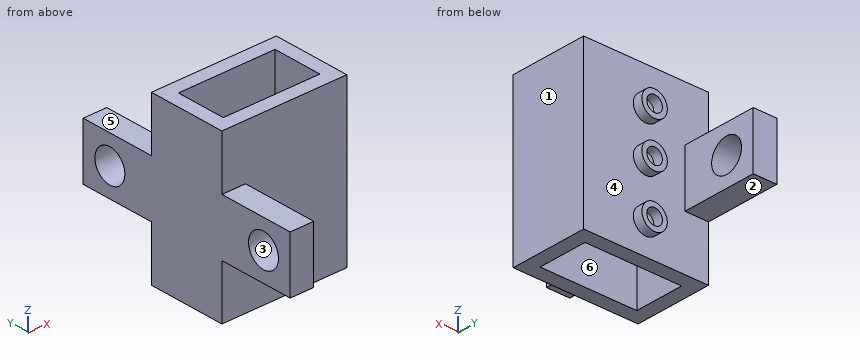
from build123d import *

# Parameters (mm, degrees)
F0_W      = 26.5
F0_H      = 35
F1_DEPTH  = 16.5
F2_W      = 20.5
F2_H      = 10.5
F3_DEPTH  = 35
F4_R      = 2.7
F4_R_2    = 1.65
F5_DEPTH  = 2
F6_W      = 5
F6_H      = 12
F7_DEPTH  = 16
F8_W      = 5
F8_H      = 12
F9_DEPTH  = 16
F10_R     = 3.5
F11_DEPTH = 5
F12_R     = 3.5
F13_DEPTH = 5


with BuildPart() as f1:
    # F0 (on Front) → F1 (new body)
    with BuildSketch(Plane.XZ):
        Rectangle(F0_W, F0_H)
    extrude(amount=F1_DEPTH)

    # F2 (on face) → F3 (cut)
    with BuildSketch(Plane.XY.offset(17.5)):
        with Locations((0, -8.25)):
            Rectangle(F2_W, F2_H)
    extrude(amount=-F3_DEPTH, mode=Mode.SUBTRACT)

    # F4 (on face) → F5 (join)
    with BuildSketch(Plane(origin=(0, 0, 0), x_dir=(-1, 0, 0), z_dir=(0, 1, 0))):
        Circle(F4_R)
        Circle(F4_R_2, mode=Mode.SUBTRACT)
        with Locations((0, 9.5)):
            Circle(F4_R)
        with Locations((0, 9.5)):
            Circle(F4_R_2, mode=Mode.SUBTRACT)
        with Locations((0, -11)):
            Circle(F4_R)
        with Locations((0, -11)):
            Circle(F4_R_2, mode=Mode.SUBTRACT)
    extrude(amount=F5_DEPTH)

    # F6 (on face) → F7 (join)
    with BuildSketch(Plane.XZ.offset(16.5)):
        with Locations((-10.75, 0)):
            Rectangle(F6_W, F6_H)
    extrude(amount=F7_DEPTH)

    # F8 (on face) → F9 (join)
    with BuildSketch(Plane(origin=(0, 0, 0), x_dir=(-1, 0, 0), z_dir=(0, 1, 0))):
        with Locations((10.75, 0)):
            Rectangle(F8_W, F8_H)
    extrude(amount=F9_DEPTH)

    # F10 (on face) → F11 (cut)
    with BuildSketch(Plane.YZ.offset(-8.25)):
        with Locations((9.75, 0)):
            Circle(F10_R)
    extrude(amount=-F11_DEPTH, mode=Mode.SUBTRACT)

    # F12 (on face) → F13 (cut)
    with BuildSketch(Plane.YZ.offset(-8.25)):
        with Locations((-26.25, 0)):
            Circle(F12_R)
    extrude(amount=-F13_DEPTH, mode=Mode.SUBTRACT)


solid = f1.part
Input: part model. Units: mm. Frame: model coordinates. Face numbers are marked on the shaded views. A direction names the side the tool comes from. Coordinates: 2 decimals unless noted, no trailing zeros. Write each loop counter-clockwise with the first axis right and the second up, starting at its lowest first coordinate (ties: lowest second). Pieces come first, ordered by that corner, then holes. Notation, with made-up numbers: M 6.25,30 L 23.25,30 A23 cw 23.25,69 Z; hole C -14.5,39 d7. An arc over 180 degrees is marked long. Answer as a JSON object with one key per item and string values. Group by question number.
(1) Section A-A on x = -9. Output: boundary loops of the cut face in (y, z), plus the area to 3 significant figures.
(2) Section B-B on z = 1. Output: boundary loops of the cut face in (x, y), plus the area to 3 significant figures.
(3) Mould query, pull axis Z, two halves, no side actions, for the marked faces 1, 2 and 3. Classes: pulls with the +Z half, pulls with the -Z half, needs draft (parallel to the pull), parting line crosses it, or undercut.
(4) Ray query, line 1 along Z through (x, y) = (0, 1.2); line 2 along Z through (x, y) = (-11.85, 9.75); line 3 along Y through (x, z) = (0, 4). Return the intervals inside material, ascending. Write a range as [from, to].
(5) Section D-D on x = -5.25. Output: boundary loops of the cut face in (y, z).
(6) Set-up query: the marked faces 4, 5 and 6. Return all of +Z, -Z, +X, -X, +Y, -Y with unobstructed straight access to the full face (end or side cutting, diameter ignored); none if empty.
(7) Section C-C on y = -9.5. Output: boundary loops of the cut face in (x, z).
(8) Contact query for flat-ended pins moving along their axis: P1, Ø4, axis at x = 10.5, z = 2, coming from the +Y side; P2, Ø5.5, axis at x = -10.5, y = -27.5, coming from the +Z side; P3, Ø5.5, axis at x = -10, y = 8, coming from the -Z side. Output: stop coordinate, or through.
Result set:
{
 "1": {"outline": "M -32.5,-6 L -16.5,-6 L -16.5,-17.5 L -13.5,-17.5 L -13.5,17.5 L -16.5,17.5 L -16.5,6 L -32.5,6 Z; M -3,-17.5 L 0,-17.5 L 0,-6 L 16,-6 L 16,6 L 0,6 L 0,17.5 L -3,17.5 Z; hole C -26.25,0 d7; hole C 9.75,0 d7", "area": "517 mm2"},
 "2": {"outline": "M -13.25,-32.5 L -8.25,-32.5 L -8.25,-29.6 L -13.25,-29.6 Z; M -13.25,-22.9 L -8.25,-22.9 L -8.25,-16.5 L 13.25,-16.5 L 13.25,0 L 2.51,0 L 2.51,2 L 1.31,2 L 1.31,0 L -1.31,0 L -1.31,2 L -2.51,2 L -2.51,0 L -8.25,0 L -8.25,6.4 L -13.25,6.4 Z; M -13.25,13.1 L -8.25,13.1 L -8.25,16 L -13.25,16 Z; hole M -10.25,-13.5 L 10.25,-13.5 L 10.25,-3 L -10.25,-3 Z", "area": "320 mm2"},
 "3": {"face 1": "needs draft", "face 2": "pulls with the -Z half", "face 3": "undercut"},
 "4": {"line 1": "z = [-13.7, -12.65], [-9.35, -8.3], [-2.7, -1.65], [1.65, 2.7], [6.8, 7.85], [11.15, 12.2]", "line 2": "z = [-6, -3.5], [3.5, 6]", "line 3": "y = [-16.5, -13.5], [-3, 0]"},
 "5": {"outline": "M -16.5,-17.5 L -13.5,-17.5 L -13.5,17.5 L -16.5,17.5 Z; M -3,-17.5 L 0,-17.5 L 0,17.5 L -3,17.5 Z"},
 "6": {"face 4": "+Y", "face 5": "+Z, +X, -X, +Y", "face 6": "+Z, -Z"},
 "7": {"outline": "M -13.25,-17.5 L -10.25,-17.5 L -10.25,17.5 L -13.25,17.5 Z; M 10.25,-17.5 L 13.25,-17.5 L 13.25,17.5 L 10.25,17.5 Z"},
 "8": {"P1": "stops at y = 0", "P2": "stops at z = 6", "P3": "stops at z = -6"}
}
